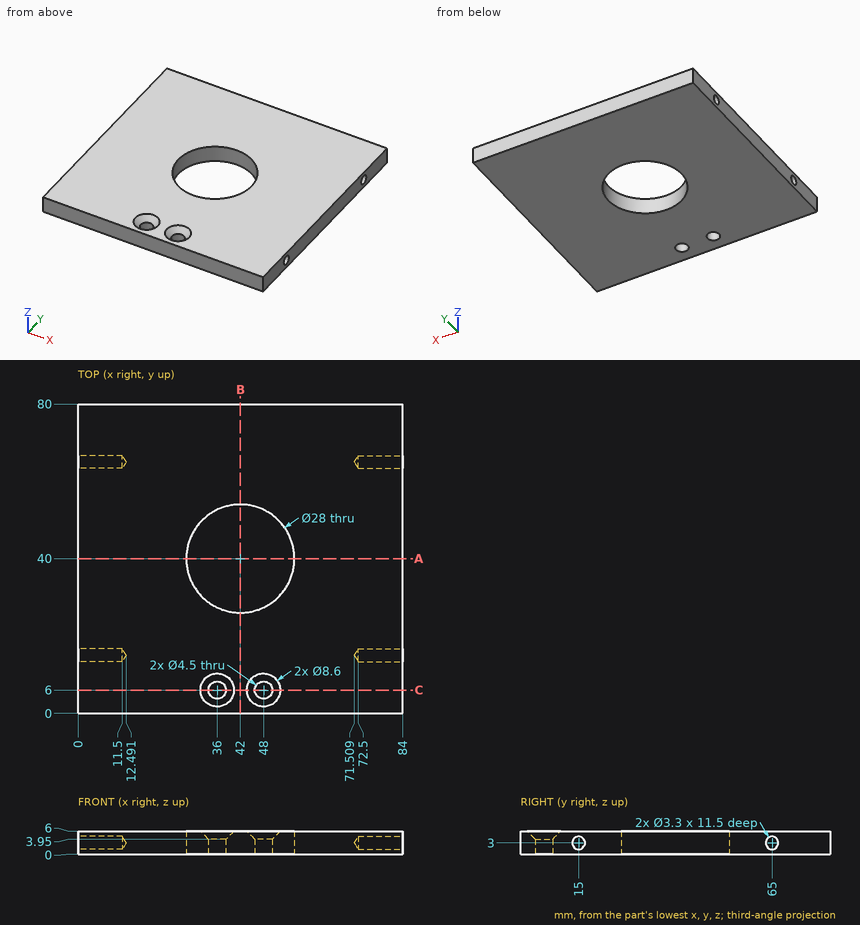
For this review, use the dimensioned drawing (mm, ordinates from the lowest corner) and the shaded views. Round coordinates to 2 decimals unless told otherwise and drop trailing zeros. Order: outer loops, then holes, each group sorted by start corner. A loop starts at its lowest first (then second) coordinate and runs counter-clockwise, first axis right, second up. Notation, with made-up numbers: (56.5, -39.5) -> (85.5, -39.5) arc R12 cw to (85.5, -23.5) -> close; hole circle Ø1 at (54, 64.5). An arc over 180 degrees is marked (long way). Write item = value, one per line. Start each with the question number.
Item 1: For line 1 along Y through (x, z) = (79.25, 3); line 2 along Z through (x, y) = (80, 15); line 3 along Y through (x, z) = (79.5, 4.15) (1 decimal), list the stretches that pass through material, from the lowest coordinate up.
Item 2: Consider section A-A on y = 40. Write out the cut boundary in (x, z), plus the area to 3 significant figures.
Item 3: Consider section C-C on y = 6. Write out the cut boundary in (x, z).
Item 4: Consider section B-B on x = 42. Write out the cut boundary in (y, z).
Item 5: Clearance check with flat-ended pins moving along their axes: pin 1 Ø7 at (x, y) = (36, 6) entering from +Z; pin 2 Ø7 at (x, y) = (48, 6) entering from -Z; pin 3 Ø2 at (y, z) = (65, 3) entering from -X; pin 4 Ø2.5 at (y, z) = (15, 3) entering from +X. State where each tip first meets the part, or that it passes through.
Conclusion:
q1.line_1 = 0 to 13.35, 16.65 to 63.35, 66.65 to 80
q1.line_2 = 0 to 1.35, 4.65 to 6
q1.line_3 = 0 to 13.8, 16.2 to 63.8, 66.2 to 80
q2.outline = (0, 0) -> (28, 0) -> (28, 6) -> (0, 6) -> close; (56, 0) -> (84, 0) -> (84, 6) -> (56, 6) -> close
q2.area = 336 mm2
q3.outline = (0, 0) -> (33.75, 0) -> (33.75, 3.95) -> (31.7, 6) -> (0, 6) -> close; (38.25, 0) -> (45.75, 0) -> (45.75, 3.95) -> (43.7, 6) -> (40.3, 6) -> (38.25, 3.95) -> close; (50.25, 0) -> (84, 0) -> (84, 6) -> (52.3, 6) -> (50.25, 3.95) -> close
q4.outline = (0, 0) -> (26, 0) -> (26, 6) -> (0, 6) -> close; (54, 0) -> (80, 0) -> (80, 6) -> (54, 6) -> close
q5.pin_1 = 5.2
q5.pin_2 = 0
q5.pin_3 = 11.89
q5.pin_4 = 72.26
